Input: part model. Units: mm. Frame: model coordinates. A direction names the side the tool comes from. Round coordinates to 2 decimals unless told otherwise and drop trailing zeros. Write each loop counter-clockwise with the first axis right and the second up, starting at its lowest first coordinate (ties: lowest second). Pieces come first, ordered by that corner, then holes. Notation, with made-up numbers: M 29.5,-26.5 L 51.5,-26.5 A20 cw 51.5,-22.5 Z; hole C 75,59 d6. An arc over 180 degrees is marked long. Answer as CSV lines item,"result". Start each with the question number.
```python
from build123d import *

# Parameters (mm, degrees)
F0_W      = 40
F0_H      = 86.76
F1_DEPTH  = 4
F2_W      = 95
F2_H      = 25
F3_DEPTH  = 27.5
F4_W      = 86.76
F4_H      = 25
F5_DEPTH  = 27.5
F6_W      = 94.977141
F6_H      = 50
F7_DEPTH  = 10
F8_R      = 5
F9_R      = 5
F10_R     = 2.5
F11_DEPTH = 10.001


with BuildPart() as f1:
    # F0 (on Top) → F1 (new body)
    with BuildSketch(Plane.XY):
        Rectangle(F0_W, F0_H)
    extrude(amount=F1_DEPTH)

    # F2 (on face) → F3 (join)
    with BuildSketch(Plane.YZ.offset(20)):
        with Locations((4.12, 12.5)):
            Rectangle(F2_W, F2_H)
    extrude(amount=F3_DEPTH)

    # F4 (on face) → F5 (join)
    with BuildSketch(Plane(origin=(-20, 0, 0), x_dir=(0, -1, 0), z_dir=(-1, 0, 0))):
        with Locations((0, 12.5)):
            Rectangle(F4_W, F4_H)
    extrude(amount=F5_DEPTH)

    # F6 (on face) → F7 (join)
    with BuildSketch(Plane(origin=(0, 43.38, 0), x_dir=(-1, 0, 0), z_dir=(0, 1, 0))):
        with Locations((-0.01143, 25)):
            Rectangle(F6_W, F6_H)
    extrude(amount=F7_DEPTH)

    # F8
    f8_edges = [f1.edges().sort_by_distance(p)[0] for p in [
        (47.5, 48.38, 50),
    ]]
    fillet(f8_edges, radius=F8_R)

    # F9
    f9_edges = [f1.edges().sort_by_distance(p)[0] for p in [
        (-47.477141, 48.38, 50),
    ]]
    fillet(f9_edges, radius=F9_R)

    # F10 (on face) → F11 (cut, through all)
    with BuildSketch(Plane.XZ.offset(-43.38)):
        with Locations((-42.477141, 45)):
            Circle(F10_R)
        with Locations((42.5, 45)):
            Circle(F10_R)
    extrude(amount=-F11_DEPTH, mode=Mode.SUBTRACT)


solid = f1.part
```
Item 1: Cut plane B-B, the plane y = 22.5. Return loops of the section in (x, z).
Item 2: Access query for faces 4 (the face through (20, -1, 15)), 5 (the face through (-34, 1, 25)), 6 (the face through (1, 53.38, 25)). Directions: +Z, -Z, +X, -X, +Y, -Y. A direction counts if a zero-diameter tool reaches every point of the face in a straight line with its end or side. Return the directions, or none.
Item 3: Cut plane D-D, the plane x = 25.5. Return loops of the section in (y, z).
Item 4: Pin query (flat end, axial travel): pin 1 Ø12 at (x, z) = (13, 34.5) entering from -Y; pin 2 Ø2 at (y, z) = (13, 27) entering from +X; pin 3 Ø22 at (x, y) = (-32, -17.5) entering from +Z. Return the tip coordinate at first contact, or that it passes through.
Item 5: Draft query along Z for faces 1 (the face through (-45.974, 48.45, 48.574)), 2 (the face through (44.81, 48.31, 44.04)), 3 (the face through (47.5, -1, 13)). Return one class per face: +Z half, -Z half, draft (parallel to the pull), parting line (faces both ways), or undercut.
Item 6: Cut plane C-C, the plane x = -11. Return loops of the section in (y, z), plus the area to 3 significant figures.
Item 7: Line query: line 1 (X direction, y = -24.5, z = 16.5); line 2 (Z direction, x = -12, y = -26); line 3 (Z direction, x = -35, y = 26.5). Output: solid intervals per line, ascending. Write a range as [from, to].
Results list:
1,outline,"M -47.5,0 L 47.5,0 L 47.5,25 L 20,25 L 20,4 L -20,4 L -20,25 L -47.5,25 Z"
2,face 4,"+Z, -Y"
2,face 5,"+Z, +X, -X, -Y"
2,face 6,"+Z, -Z, +X, -X, +Y"
3,outline,"M -43.38,0 L 53.38,0 L 53.38,50 L 43.38,50 L 43.38,25 L -43.38,25 Z"
4,pin 1,"y = 43.38"
4,pin 2,"through"
4,pin 3,"z = 25"
5,face 1,"+Z half"
5,face 2,"undercut"
5,face 3,"draft"
6,outline,"M -43.38,0 L 53.38,0 L 53.38,50 L 43.38,50 L 43.38,4 L -43.38,4 Z"
6,area,"847 mm²"
7,line 1,"[-47.5, -20], [20, 47.5]"
7,line 2,"[0, 4]"
7,line 3,"[0, 25]"
